```python
from build123d import *

# Parameters (mm, degrees)
EXTRUDE_1_DEPTH        = 12
FILLET_1_R             = 5
HOLE_WIZARD_M5_1_D     = 4.2
HOLE_WIZARD_M5_1_DEPTH = 12.4
HOLE_WIZARD_M5_1_TIP   = 1.2618073
HOLE_WIZARD_M5_2_D     = 4.2
HOLE_WIZARD_M5_2_DEPTH = 12.4
HOLE_WIZARD_M5_2_TIP   = 1.2618073


with BuildPart() as part:
    # 草图1 → 凸台-拉伸1 (new body)
    with BuildSketch(Plane.XY):
        Polygon((0, 0), (-45, 0), (-45, 33), (-80, 33), (-80, 100), (0, 100), align=None)
    extrude(amount=EXTRUDE_1_DEPTH)

    # 圆角1
    fillet_1_edges = [part.edges().sort_by_distance(p)[0] for p in [
        (-45, 33, 6),
    ]]
    fillet(fillet_1_edges, radius=FILLET_1_R)

    # M5 螺纹孔1
    with Locations(Plane.XZ):
        with Locations((-6, 6), (-21, 6)):
            Hole(HOLE_WIZARD_M5_1_D / 2, depth=HOLE_WIZARD_M5_1_DEPTH)
            with Locations((0, 0, -(HOLE_WIZARD_M5_1_DEPTH + HOLE_WIZARD_M5_1_TIP / 2))):  # 118° drill point
                Cone(0, HOLE_WIZARD_M5_1_D / 2, HOLE_WIZARD_M5_1_TIP, mode=Mode.SUBTRACT)

    # M5 螺纹孔2
    with Locations(Plane(origin=(0, 100, 0), x_dir=(-1, 0, 0), z_dir=(0, 1, 0))):
        with Locations((38, 6), (64, 6)):
            Hole(HOLE_WIZARD_M5_2_D / 2, depth=HOLE_WIZARD_M5_2_DEPTH)
            with Locations((0, 0, -(HOLE_WIZARD_M5_2_DEPTH + HOLE_WIZARD_M5_2_TIP / 2))):  # 118° drill point
                Cone(0, HOLE_WIZARD_M5_2_D / 2, HOLE_WIZARD_M5_2_TIP, mode=Mode.SUBTRACT)


solid = part.part
```
Input: part model. Units: mm. Frame: model coordinates. A direction names the side the tool comes from. Coordinates: 2 decimals unless noted, no trailing zeros. Write each loop counter-clockwise with the first axis right and the second up, starting at its lowest first coordinate (ties: lowest second). Pieces come first, ordered by that corner, then holes.
1) Pin query (flat end, axial travel): pin 1 Ø3.5 at (x, z) = (-21, 6) entering from -Y; pin 2 Ø6 at (x, z) = (-61, 9.5) entering from -Y; pin 3 Ø4 at (x, z) = (-64, 6) entering from +Y. Return the tip coordinate at first contact, or that it passes through.
2) Mould query, pull axis Z, two halves, no side actions, for faces 4 (the flat face through (-45, 14, 6)), 5 (the flat face through (-39, 62, 0)), 6 (the cylindrical face through (-5.727, 6.287, 8.082)), 7 (the cylindrical face through (-23.003, 6.287, 6.631)). Classes: pulls with the +Z half, pulls with the -Z half, needs draft (parallel to the pull), parting line crosses it, or undercut.
3) Material intervals for line 1 along X through (y, z) = (91.25, 6); line 2 along X through (y, z) = (9.5, 6); line 3 along Z through (x, y) = (-21, 9.5), sorted ascending.
4) Section A-A on x = -68.5. Output: boundary loops of the cut face in (y, z), and give its area (3 significant figures).
5) Set-up query: faces 1 (the flat face through (0, 51, 6)), 2 (the flat face through (-65, 33, 6)), 3 (the cylindrical face through (-39.548, 93.713, 7.419)). Return all of +Z, -Z, +X, -X, +Y, -Y with unobstructed straight access to the full face (end or side cutting, diameter ignored); none if empty.
6) Section B-B on y = 15.5. Output: boundary loops of the cut face in (x, z).
Check result:
1. pin 1: stops at y = 12.61
1. pin 2: stops at y = 33
1. pin 3: stops at y = 87.54
2. face 4: needs draft
2. face 5: pulls with the -Z half
2. face 6: undercut
2. face 7: undercut
3. line 1: x = -80 to -66.1, -61.9 to -40.1, -35.9 to 0
3. line 2: x = -45 to -23.1, -18.9 to -8.1, -3.9 to 0
3. line 3: z = 0 to 3.9, 8.1 to 12
4. outline: (33, 0) - (100, 0) - (100, 12) - (33, 12) - close
4. area: 804 mm2
5. face 1: +Z, -Z, +X, +Y, -Y
5. face 2: +Z, -Z, -X, -Y
5. face 3: +Y
6. outline: (-45, 0) - (0, 0) - (0, 12) - (-45, 12) - close
